from build123d import *

# Parameters (mm, degrees)
F0_W      = 88
F0_H      = 15.5
F1_DEPTH  = 2.1
F2_W      = 15.5
F2_H      = 2.1
F3_DEPTH  = 33
F4_W      = 88
F4_H      = 31
F5_DEPTH  = 2.1
F6_W      = 15.5
F6_H      = 2.1
F7_DEPTH  = 33
F8_W      = 88
F8_H      = 31
F9_DEPTH  = 2.21
F10_W     = 15.5
F10_H     = 2.1
F10_W_2   = 2.1
F10_H_2   = 28.9
F11_DEPTH = 33
F12_W     = 88
F12_H     = 31
F13_DEPTH = 2.1
F14_W     = 88
F14_H     = 31
F14_W_2   = 83.8
F14_H_2   = 26.8
F15_DEPTH = 10
F16_R     = 1
F17_DEPTH = 2.1
F18_W     = 31
F18_H     = 2
F19_DEPTH = 2.1


with BuildPart() as f1:
    # F0 (on Top) → F1 (new body)
    with BuildSketch(Plane.XY):
        with Locations((0, -7.75)):
            Rectangle(F0_W, F0_H)
        with Locations((0, -23.25)):
            Rectangle(F0_W, F0_H)
    extrude(amount=-F1_DEPTH)

    # F2 (on face) → F3 (join)
    with BuildSketch(Plane.XY):
        Polygon((-26.4, 0), (-28.5, 0), (-28.5, -2.1), (-28.5, -28.9), (-28.5, -31), (-26.4, -31), align=None)
        with Locations((-36.25, -1.05)):
            Rectangle(F2_W, F2_H)
        with Locations((-36.25, -29.95)):
            Rectangle(F2_W, F2_H)
        Polygon((28.5, 0), (26.4, 0), (26.4, -31), (28.5, -31), (28.5, -28.9), (28.5, -2.1), align=None)
        with Locations((36.25, -1.05)):
            Rectangle(F2_W, F2_H)
        with Locations((36.25, -29.95)):
            Rectangle(F2_W, F2_H)
    extrude(amount=F3_DEPTH)

    # F4 (on face) → F5 (join)
    with BuildSketch(Plane.XY.offset(33)):
        with Locations((0, -15.5)):
            Rectangle(F4_W, F4_H)
    extrude(amount=F5_DEPTH)

    # F6 (on face) → F7 (join)
    with BuildSketch(Plane.XY.offset(35.1)):
        Polygon((-26.4, 0), (-28.5, 0), (-28.5, -2.1), (-28.5, -28.9), (-28.5, -31), (-26.4, -31), align=None)
        with Locations((-36.25, -1.05)):
            Rectangle(F6_W, F6_H)
        with Locations((-36.25, -29.95)):
            Rectangle(F6_W, F6_H)
        Polygon((28.5, 0), (26.4, 0), (26.4, -31), (28.5, -31), (28.5, -28.9), (28.5, -2.1), align=None)
        with Locations((36.25, -29.95)):
            Rectangle(F6_W, F6_H)
        with Locations((36.25, -1.05)):
            Rectangle(F6_W, F6_H)
    extrude(amount=F7_DEPTH)

    # F8 (on face) → F9 (join)
    with BuildSketch(Plane.XY.offset(68.1)):
        with Locations((0, -15.5)):
            Rectangle(F8_W, F8_H)
    extrude(amount=F9_DEPTH)

    # F10 (on face) → F11 (join)
    with BuildSketch(Plane.XY.offset(70.31)):
        with Locations((-36.25, -1.05)):
            Rectangle(F10_W, F10_H)
        Polygon((28.5, -28.9), (28.5, -31), (44, -31), (44, -28.9), (41.9, -28.9), align=None)
        with Locations((-36.25, -29.95)):
            Rectangle(F10_W, F10_H)
        Polygon((-26.4, 0), (-28.5, 0), (-28.5, -2.1), (-28.5, -28.9), (-28.5, -31), (-26.4, -31), align=None)
        Polygon((28.5, 0), (26.4, 0), (26.4, -31), (28.5, -31), (28.5, -28.9), align=None)
        with Locations((42.95, -14.45)):
            Rectangle(F10_W_2, F10_H_2)
    extrude(amount=F11_DEPTH)

    # F12 (on face) → F13 (join)
    with BuildSketch(Plane.XY.offset(103.31)):
        with Locations((0, -15.5)):
            Rectangle(F12_W, F12_H)
    extrude(amount=F13_DEPTH)

    # F14 (on face) → F15 (join)
    with BuildSketch(Plane.XY.offset(105.41)):
        with Locations((0, -15.5)):
            Rectangle(F14_W, F14_H)
        with Locations((0, -15.5)):
            Rectangle(F14_W_2, F14_H_2, mode=Mode.SUBTRACT)
    extrude(amount=F15_DEPTH)

    # F16 (on face) → F17 (cut)
    with BuildSketch(Plane.XZ.offset(31)):
        with Locations((-36, 107.41)):
            Circle(F16_R)
        with Locations((36, 107.41)):
            Circle(F16_R)
    extrude(amount=-F17_DEPTH, mode=Mode.SUBTRACT)

    # F18 (on face) → F19 (cut)
    with BuildSketch(Plane(origin=(26.4, 0, 0), x_dir=(0, -1, 0), z_dir=(-1, 0, 0))):
        with Locations((15.5, 86.81)):
            Rectangle(F18_W, F18_H)
        with Locations((15.5, 51.71)):
            Rectangle(F18_W, F18_H)
        with Locations((15.5, 16.61)):
            Rectangle(F18_W, F18_H)
    extrude(amount=-F19_DEPTH, mode=Mode.SUBTRACT)


solid = f1.part
Design review of the part built by this model. Coordinates are the model's own, in mm. A direction names the side the tool comes from. Coordinates: 2 decimals unless noted, no trailing zeros. Loops run counter-clockwise (first coordinate to the right, second up) from the corner with the lowest first, then second, coordinate; pieces in that order, holes last.
Item 1: Draft analysis for pull direction X (two halves, no side actions). For faces 1 (the flat face through (-36, -15, 33)), 2 (the flat face through (28.5, -16, 60)), 3 (the flat face through (-1, -15, 105.41)), 4 (the flat face through (0, -15, 0)), state which applies: pulls with the +X half, pulls with the -X half, needs draft (parallel to the pull), parting line crosses it, or undercut.
Completed:
face 1: needs draft
face 2: pulls with the +X half
face 3: undercut
face 4: undercut
Item 2: Wall thickness on L1, parallel to X at y = -29.7, z = 107.41; L2, parallel to Z at x = 32, y = -24; L3, parallel to Z at x = -0.5, y = -2: over which ranges is each line inside the solid? List them lowest first.
Completed:
L1: x = -44 to -37, -35 to 35, 37 to 44
L2: z = -2.1 to 0, 33 to 35.1, 68.1 to 70.31, 103.31 to 105.41
L3: z = -2.1 to 0, 33 to 35.1, 68.1 to 70.31, 103.31 to 115.41
Item 3: Clearance check with flat-ended pins moving along their axes: pin 1 (3 mm diameter, centred on x = 12.5, y = -4, fed in from +Z); pin 2 (17 mm diameter, centred on y = -18.5, z = 94, fed in from -X). State where each tip first meets the part, or that it passes through.
Completed:
pin 1: stops at z = 105.41
pin 2: stops at x = -28.5
Item 4: Add section A-A (x = -15). Write out the cut boundary in (y, z), and give its area (3 significant figures).
Completed:
outline: (-31, -2.1) - (0, -2.1) - (0, 0) - (-31, 0) - close; (-31, 33) - (0, 33) - (0, 35.1) - (-31, 35.1) - close; (-31, 68.1) - (0, 68.1) - (0, 70.31) - (-31, 70.31) - close; (-31, 103.31) - (0, 103.31) - (0, 115.41) - (-2.1, 115.41) - (-2.1, 105.41) - (-28.9, 105.41) - (-28.9, 115.41) - (-31, 115.41) - close
area: 306 mm2
Item 5: For faces 5 (the flat face through (-1, -15, -2.1)), 6 (the flat face through (-28.5, -15, 16)), 7 (the flat face through (36, -28.9, 16)), 8 (the flat face through (26.4, -15, 78)), 9 (the flat face through (-41.9, -16, 110)), list the 3-axis set-ups (+Z, -Z, +X, -X, +Y, -Y) from which the entire face can be reached by the end or side of a thin tool; tool diameter is ignored.
Completed:
face 5: -Z, +X, -X, +Y, -Y
face 6: -X
face 7: +X
face 8: +Y, -Y
face 9: +Z
Item 6: Add section B-B (z = 40). Write out the cut boundary in (x, y).
Completed:
outline: (-44, -31) - (-26.4, -31) - (-26.4, 0) - (-44, 0) - (-44, -2.1) - (-28.5, -2.1) - (-28.5, -28.9) - (-44, -28.9) - close; (26.4, -31) - (44, -31) - (44, -28.9) - (28.5, -28.9) - (28.5, -2.1) - (44, -2.1) - (44, 0) - (26.4, 0) - close
Item 7: Add section C-C (x = 31). Write out the cut boundary in (y, z).
Completed:
outline: (-31, -2.1) - (0, -2.1) - (0, 70.31) - (-28.9, 70.31) - (-28.9, 103.31) - (0, 103.31) - (0, 115.41) - (-2.1, 115.41) - (-2.1, 105.41) - (-28.9, 105.41) - (-28.9, 115.41) - (-31, 115.41) - close; hole (-28.9, 0) - (-2.1, 0) - (-2.1, 33) - (-28.9, 33) - close; hole (-28.9, 35.1) - (-2.1, 35.1) - (-2.1, 68.1) - (-28.9, 68.1) - close
